Part model, mm, in its own coordinate system. A direction names the side the tool comes from. Round coordinates to 2 decimals unless told otherwise and drop trailing zeros. Loops run counter-clockwise (first coordinate to the right, second up) from the corner with the lowest first, then second, coordinate; pieces in that order, holes last. Notation, with made-up numbers: (-32.5, 16) - (26.5, 16) arc R24 ccw to (26.5, 42) - close; hole circle Ø9 at (53.25, -10). An arc over 180 degrees is marked (long way). Write each question's results on one line, items separated by ' | '. Start each with the question number.
(1) Cut at B-B, the plane x = -6. List the corners of the cut face in (y, z).
(2) Drill centre lines: L1, parallel to Y at x = -47, z = -1; L2, parallel to X at y = -0.75, z = -12.5; L3, parallel to X at y = 15.25, z = -3. Where is each one in solid material? Low to high.
(3) Cut at C-C, the plane x = 53.5. List the corners of the cut face in (y, z), then the cut area to 3 significant figures.
(4) Cut at A-A, the plane y = 20.5. List the corners of the cut face in (x, z), then the cut area to 3 significant figures.
(5) Tool access for faces 1 (the face through (76, 22, 0)), 2 (the face through (48.81, 13.48, -0.38)), 3 (the face through (77.797, 13.141, 0.07)), 4 (the face through (51, 13, 5)), 5 (the face through (18.5, -1, -11)): list every direction of +Z, -Z, +X, -X, +Y, -Y with a clear straight run to the whole face (end or side of a thin tool).
(6) Mould opens along Z. For faces 6 (the face through (0.66, -1.479, -14.985)), 7 (the face through (-51, 13, -5)), 8 (the face through (13.8, -2.3, -12.7)), 9 (the face through (59, 15, 0)) say: released by +Z, released by -Z, zero draft, split by the parting line, or undercut.
(7) Flat gauge pins, fed straight in: P1, Ø1.5, axis at x = -52, z = 0, coming from the +Y side; P2, Ø4.5, axis at x = -14.32, z = 14.32, coming from the +Y side; P3, Ø11, axis at x = -57.5, z = -0.5, coming from the -Y side. Where does each tip first touch, or does it go through?
from build123d import *

# Parameters (mm, degrees)
SKETCH_1_W                  = 37
SKETCH_1_H                  = 37
SKETCH_1_R                  = 15
SKETCH_1_R_2                = 1.65
SM_BASE_FLANGE_1_DEPTH      = 3
FILLET_1_R                  = 3
SKETCH_6_W                  = 56.5
SKETCH_6_H                  = 10
EXTRUDE_1_DEPTH             = 3
OTHER_START                 = -5
OTHER_1_DEPTH               = 10
OTHER_1_2_DEPTH             = 10
OTHER_2_DEPTH               = 10
OTHER_2_2_DEPTH             = 10
SM_EDGE_FLANGE_1_DEPTH      = 10
SM_EDGE_FLANGE_2_DEPTH      = 10
SKETCH_18_R                 = 1
CUT_EXTRUDE_2_DEPTH         = 10
HOLE_WIZARD_M3_2_AT_2_COUNT = 2
HOLE_WIZARD_M3_2_AT_2_PITCH = 28.637824638
HOLE_WIZARD_M3_2_AT_3_COUNT = 2
HOLE_WIZARD_M3_2_AT_3_PITCH = 40.5
HOLE_WIZARD_M3_2_AT_4_COUNT = 2
HOLE_WIZARD_M3_2_AT_4_PITCH = 28.637824638
HOLE_WIZARD_M3_2_2_D        = 2.5
FILLET_2_R                  = 2
FILLET_3_R                  = 1


# Read off the part's stored shape, not the designer's step: 转折1, 转折2
# Sheet-metal steps are written as plain solids
with BuildPart() as part:
    # Sketch 1 → 基体-法兰1 (new body)
    with BuildSketch(Plane(origin=(0, 0, 0), x_dir=(1, 0, 0), z_dir=(0, 1, 0))):
        Rectangle(SKETCH_1_W, SKETCH_1_H)
        with Locations(Location((0, 0, 0), (0, 0, 270))):
            Circle(SKETCH_1_R, mode=Mode.SUBTRACT)
        with Locations(Location((-14.318912319, 14.318912319, 0), (0, 0, 270))):
            Circle(SKETCH_1_R_2, mode=Mode.SUBTRACT)
        with Locations(Location((14.318912319, 14.318912319, 0), (0, 0, 270))):
            Circle(SKETCH_1_R_2, mode=Mode.SUBTRACT)
        with Locations(Location((14.318912319, -14.318912319, 0), (0, 0, 270))):
            Circle(SKETCH_1_R_2, mode=Mode.SUBTRACT)
        with Locations(Location((-14.318912319, -14.318912319, 0), (0, 0, 270))):
            Circle(SKETCH_1_R_2, mode=Mode.SUBTRACT)
    extrude(amount=-SM_BASE_FLANGE_1_DEPTH)

    # 圆角1
    fillet_1_edges = [part.edges().sort_by_distance(p)[0] for p in [
        (18.5, -1.5, 18.5),
        (-18.5, -1.5, 18.5),
        (-18.5, -1.5, -18.5),
        (18.5, -1.5, -18.5),
    ]]
    fillet(fillet_1_edges, radius=FILLET_1_R)

    # 草图6 → 凸台-拉伸1 (add)
    with BuildSketch(Plane(origin=(0, 0, 0), x_dir=(1, 0, 0), z_dir=(0, 1, 0))):
        with Locations((-46.75, 0)):
            Rectangle(SKETCH_6_W, SKETCH_6_H)
        with Locations((46.75, 0)):
            Rectangle(SKETCH_6_W, SKETCH_6_H)
    extrude(amount=-EXTRUDE_1_DEPTH)

    # Other 1 outline → Other 1 (cut)
    with BuildSketch(Plane.XY.offset(OTHER_START)):
        with BuildLine():
            ThreePointArc((-26.972836905, -3), (-29.085928213, -2.531538935), (-30.80305912, -1.213938048))
            Line((-30.80305912, -1.213938048), (-31.821674088, 0))
            Line((-31.821674088, 0), (-75, 0))
            Line((-75, 0), (-75, -3))
            Line((-75, -3), (-26.972836905, -3))
        make_face()
    extrude(amount=OTHER_1_DEPTH, mode=Mode.SUBTRACT)

    # Other 1 2 outline → Other 1 2 (add)
    with BuildSketch(Plane.XY.offset(OTHER_START)):
        with BuildLine():
            Line((-41.291396093, 11.285575219), (-31.821674088, 0))
            Line((-31.821674088, 0), (-26.972836905, 0))
            ThreePointArc((-26.972836905, 0), (-27.818073428, 0.187384426), (-28.504925791, 0.714424781))
            Line((-28.504925791, 0.714424781), (-38.993262764, 13.213938048))
            ThreePointArc((-38.993262764, 13.213938048), (-40.710393671, 14.531538935), (-42.823484979, 15))
            Line((-42.823484979, 15), (-75, 15))
            Line((-75, 15), (-75, 12))
            Line((-75, 12), (-42.823484979, 12))
            ThreePointArc((-42.823484979, 12), (-41.978248456, 11.812615574), (-41.291396093, 11.285575219))
        make_face()
    extrude(amount=OTHER_1_2_DEPTH)

    # Other 2 outline → Other 2 (cut)
    with BuildSketch(Plane.XY.offset(OTHER_START)):
        with BuildLine():
            Line((75, 0), (31.821674088, 0))
            Line((31.821674088, 0), (30.80305912, -1.213938048))
            ThreePointArc((30.80305912, -1.213938048), (29.085928213, -2.531538935), (26.972836905, -3))
            Line((26.972836905, -3), (75, -3))
            Line((75, -3), (75, 0))
        make_face()
    extrude(amount=OTHER_2_DEPTH, mode=Mode.SUBTRACT)

    # Other 2 2 outline → Other 2 2 (add)
    with BuildSketch(Plane.XY.offset(OTHER_START)):
        with BuildLine():
            Line((42.823484979, 12), (75, 12))
            Line((75, 12), (75, 15))
            Line((75, 15), (42.823484979, 15))
            ThreePointArc((42.823484979, 15), (40.710393671, 14.531538935), (38.993262764, 13.213938048))
            Line((38.993262764, 13.213938048), (28.504925791, 0.714424781))
            ThreePointArc((28.504925791, 0.714424781), (27.818073428, 0.187384426), (26.972836905, 0))
            Line((26.972836905, 0), (31.821674088, 0))
            Line((31.821674088, 0), (41.291396093, 11.285575219))
            ThreePointArc((41.291396093, 11.285575219), (41.978248456, 11.812615574), (42.823484979, 12))
        make_face()
    extrude(amount=OTHER_2_2_DEPTH)

    # 边线-法兰1 section (across the edge) → 边线-法兰1 (add)
    with BuildSketch(Plane(origin=(76, 15, 5), x_dir=(-1, 0, 0), z_dir=(0, 0, -1))):
        with BuildLine():
            Line((-3, 1), (-3, 12))
            Line((-3, 12), (0, 12))
            Line((0, 12), (0, 1))
            ThreePointArc((0, 1), (0.292893219, 0.292893219), (1, 0))
            Line((1, 0), (1, -3))
            ThreePointArc((1, -3), (-1.828427125, -1.828427125), (-3, 1))
        make_face()
    extrude(amount=SM_EDGE_FLANGE_1_DEPTH)

    # 边线-法兰2 section (across the edge) → 边线-法兰2 (add)
    with BuildSketch(Plane(origin=(-76, 15, -5), x_dir=(1, 0, 0), z_dir=(0, 0, 1))):
        with BuildLine():
            Line((-3, 1), (-3, 12))
            Line((-3, 12), (0, 12))
            Line((0, 12), (0, 1))
            ThreePointArc((0, 1), (0.292893219, 0.292893219), (1, 0))
            Line((1, 0), (1, -3))
            ThreePointArc((1, -3), (-1.828427125, -1.828427125), (-3, 1))
        make_face()
    extrude(amount=SM_EDGE_FLANGE_2_DEPTH)

    # 草图18 → 切除-拉伸2 (cut)
    with BuildSketch(Plane.ZX.offset(15)):
        with Locations(Location((0, 50, 0), (0, 0, 270))):
            Circle(SKETCH_18_R)
        with Locations(Location((0, 70, 0), (0, 0, 270))):
            Circle(SKETCH_18_R)
        with Locations((0, -70)):
            Circle(SKETCH_18_R)
        with Locations((0, -50)):
            Circle(SKETCH_18_R)
    extrude(amount=-CUT_EXTRUDE_2_DEPTH, mode=Mode.SUBTRACT)

    # 草图24 → Hole Wizard M3 _2 (revolve, cut)
    with BuildSketch(Plane(origin=(-14.318912319, 0, -14.318912319), x_dir=(0, 0, 1), z_dir=(1, 0, 0))):
        Polygon((0, 0), (0, 3), (1.7, 3), (1.7, 1.6), (3.3, 0), align=None)
    hole_wizard_m3_2 = revolve(axis=Axis((-14.318912319, 6.35, -14.318912319), (0, -1, 0)), mode=Mode.SUBTRACT)

    # Hole Wizard M3 _2 at 2: Hole Wizard M3 _2 ×2
    with Locations(*[(i * HOLE_WIZARD_M3_2_AT_2_PITCH, 0, 0) for i in range(1, HOLE_WIZARD_M3_2_AT_2_COUNT)]):
        add(hole_wizard_m3_2, mode=Mode.SUBTRACT)

    # Hole Wizard M3 _2 at 3: Hole Wizard M3 _2 ×2
    with Locations(*[Vector(0.7071067811865451, 0, 0.70710678118655) * (i * HOLE_WIZARD_M3_2_AT_3_PITCH) for i in range(1, HOLE_WIZARD_M3_2_AT_3_COUNT)]):
        add(hole_wizard_m3_2, mode=Mode.SUBTRACT)

    # Hole Wizard M3 _2 at 4: Hole Wizard M3 _2 ×2
    with Locations(*[(0, 0, i * HOLE_WIZARD_M3_2_AT_4_PITCH) for i in range(1, HOLE_WIZARD_M3_2_AT_4_COUNT)]):
        add(hole_wizard_m3_2, mode=Mode.SUBTRACT)

    # Hole Wizard M3 _2 2 (through all)
    with Locations(Plane(origin=(0, 15, 0), x_dir=(1, 0, 0), z_dir=(0, 1, 0))):
        with Locations((-70, 0), (-50, 0), (50, 0), (70, 0)):
            Hole(HOLE_WIZARD_M3_2_2_D / 2)

    # 圆角2
    fillet_2_edges = [part.edges().sort_by_distance(p)[0] for p in [
        (77.5, 27, 5),
        (77.5, 27, -5),
        (-77.5, 27, -5),
        (-77.5, 27, 5),
    ]]
    fillet(fillet_2_edges, radius=FILLET_2_R)

    # 圆角3
    fillet_3_edges = [part.edges().sort_by_distance(p)[0] for p in [
        (18.5, -1.5, -5),
        (18.5, -1.5, 5),
        (-18.5, -1.5, -5),
        (-18.5, -1.5, 5),
    ]]
    fillet(fillet_3_edges, radius=FILLET_3_R)


solid = part.part
A:
1) outline: (-3, -18.5) - (0, -18.5) - (0, -13.75) - (-3, -13.75) - close; (-3, 13.75) - (0, 13.75) - (0, 18.5) - (-3, 18.5) - close
2) L1: 12 to 15 | L2: -18.5 to -16.11, -12.53 to -8.29, 8.29 to 12.53, 16.11 to 18.5 | L3: -78.93 to -75.66, 75.66 to 78.93
3) outline: (12, -5) - (15, -5) - (15, 5) - (12, 5) - close | area: 30.0 mm2
4) outline: (-79, -5) - (-76, -5) - (-76, 5) - (-79, 5) - close; (76, -5) - (79, -5) - (79, 5) - (76, 5) - close | area: 60.0 mm2
5) face 1: +Z, -Z, +Y | face 2: +Y, -Y | face 3: +Z, -Z, +X, -Y | face 4: +Z, +X, +Y, -Y | face 5: -Z, +X, +Y, -Y
6) face 6: undercut | face 7: released by -Z | face 8: undercut | face 9: zero draft
7) P1: y = 15 | P2: y = -1.05 | P3: y = 12
